from build123d import *

# Parameters (mm, degrees)
ESBO_O1_R                = 3
ESBO_O1_R_2              = 1.5
RESSALTO_EXTRUS_O2_DEPTH = 6


with BuildPart() as part:
    # Esboço1 → Ressalto-extrusão2 (new body)
    with BuildSketch(Plane.XY):
        with BuildLine():
            Line((5, 50), (28, 50))
            ThreePointArc((28, 50), (31.535533906, 48.535533906), (33, 45))
            Line((33, 45), (33, -20))
            ThreePointArc((33, -20), (31.535533906, -23.535533906), (28, -25))
            Line((28, -25), (5, -25))
            ThreePointArc((5, -25), (1.464466094, -23.535533906), (0, -20))
            Line((0, -20), (0, 45))
            ThreePointArc((0, 45), (1.464466094, 48.535533906), (5, 50))
        make_face()
        with Locations((25, 40)):
            Circle(ESBO_O1_R, mode=Mode.SUBTRACT)
        with Locations((25.5, -17)):
            Circle(ESBO_O1_R_2, mode=Mode.SUBTRACT)
        with Locations((7.5, -17)):
            Circle(ESBO_O1_R_2, mode=Mode.SUBTRACT)
        with BuildLine():
            ThreePointArc((6, 40), (11.564971157, 26.564971157), (25, 21))
            ThreePointArc((25, 21), (28, 24), (25, 27))
            ThreePointArc((25, 27), (15.807611845, 30.807611845), (12, 40))
            ThreePointArc((12, 40), (9, 43), (6, 40))
        make_face(mode=Mode.SUBTRACT)
    extrude(amount=RESSALTO_EXTRUS_O2_DEPTH)


solid = part.part
Check sheet for the modelled part. Datum: model origin and axes. Units: mm. A direction names the side the tool comes from. Round coordinates to 2 decimals unless told otherwise and drop trailing zeros. Order: outer loops, then holes, each group sorted by start corner. A loop starts at its lowest first (then second) coordinate and runs counter-clockwise, first axis right, second up.
Q1. Cross-section at D-D, the plane x = 7.5. Enter the section's corners in (y, z), plus the area to 3 significant figures.
Filled sheet:
outline: (-25, 0) - (-18.5, 0) - (-18.5, 6) - (-25, 6) - close; (-15.5, 0) - (32.6, 0) - (32.6, 6) - (-15.5, 6) - close; (42.6, 0) - (50, 0) - (50, 6) - (42.6, 6) - close
area: 372 mm2
Q2. Cross-section at C-C, the plane x = 18. Enter the section's corners in (y, z).
Filled sheet:
outline: (-25, 0) - (22.34, 0) - (22.34, 6) - (-25, 6) - close; (29.05, 0) - (50, 0) - (50, 6) - (29.05, 6) - close
Q3. Cross-section at B-B, the plane z = 2.8. Enter the section's corners in (x, y), plus the area to 3 significant figures.
Filled sheet:
outline: (0, -20) arc R5 ccw to (5, -25) - (28, -25) arc R5 ccw to (33, -20) - (33, 45) arc R5 ccw to (28, 50) - (5, 50) arc R5 ccw to (0, 45) - close; hole circle Ø3 at (7.5, -17); hole (6, 40) arc R19 ccw to (25, 21) arc R3 ccw to (25, 27) arc R13 cw to (12, 40) arc R3 ccw to start; hole circle Ø6 at (25, 40); hole circle Ø3 at (25.5, -17)
area: 2,230 mm2
Q4. Set-up check for faces 1 (the face through (28, 24, 3)), 2 (the face through (0, 12, 3)): record each of +Z, -Z, +X, -X, +Y, -Y from which the full face is reachable in a straight line by a thin tool's end or side.
Filled sheet:
face 1: +Z, -Z
face 2: +Z, -Z, -X, +Y, -Y
Q5. Cross-section at A-A, the plane y = -17. Enter the section's corners in (x, z).
Filled sheet:
outline: (0, 0) - (6, 0) - (6, 6) - (0, 6) - close; (9, 0) - (24, 0) - (24, 6) - (9, 6) - close; (27, 0) - (33, 0) - (33, 6) - (27, 6) - close
Q6. Scan lines: L1, parallel to Y at x = 25, z = 3.95; L2, parallel to Y at x = 25.5, z = 4.65; L3, parallel to Y at x = 7.5, z = 1.35. Record each from-to range of solid material in increasing order.
Filled sheet:
L1: y = -25 to -18.41, -15.59 to 21, 27 to 37, 43 to 50
L2: y = -25 to -18.5, -15.5 to 21.04, 26.96 to 37.04, 42.96 to 50
L3: y = -25 to -18.5, -15.5 to 32.6, 42.6 to 50
Q7. Draft check along X on faces 3 (the face through (6.39, -15.99, 2.96)), 4 (the face through (32, -23, 3)), 5 (the face through (17, -25, 3)). Enter one of: pulls with the +X half, pulls with the -X half, needs draft (parallel to the pull), parting line crosses it, or undercut.
Filled sheet:
face 3: undercut
face 4: pulls with the +X half
face 5: needs draft
